The model under review builds one solid part; all positions refer to its coordinate system, in mm. A direction names the side the tool comes from. Round coordinates to 2 decimals unless told otherwise and drop trailing zeros. Order: outer loops, then holes, each group sorted by start corner. A loop starts at its lowest first (then second) coordinate and runs counter-clockwise, first axis right, second up.
Autodesk Inventor part; units mm, degrees
ref_plane "YZ Plane" through (0, 0, 0) normal (1, 0, 0) x (0, 1, 0)
ref_plane "XZ Plane" through (0, 0, 0) normal (0, 1, 0) x (-1, 0, 0)
ref_plane "XY Plane" through (0, 0, 0) normal (0, 0, 1) x (1, 0, 0)
sketch "Sketch1" plane through (0, 0, 0) normal (0, 0, 1) x (1, 0, 0)
  line L0 (-21, 21) -> (21, 21) construction
  line L1 (21, 21) -> (21, -21) construction
  line L2 (21, -21) -> (-21, -21) construction
  line L3 (-21, -21) -> (-21, 21) construction
  line L4 (-21, 16.9706) -> (-21, -16.9706)
  line L5 (-16.9706, -21) -> (16.9706, -21)
  line L6 (21, -16.9706) -> (21, 16.9706)
  line L7 (16.9706, 21) -> (-16.9706, 21)
  arc A0 (-16.9706, 21) -> (-21, 16.9706) centre (0, 0) ccw
  arc A1 (-21, -16.9706) -> (-16.9706, -21) centre (0, 0) ccw
  arc A2 (16.9706, -21) -> (21, -16.9706) centre (0, 0) ccw
  arc A3 (21, 16.9706) -> (16.9706, 21) centre (0, 0) ccw
  dimension "d0" = 42
  dimension "d3" = 27
extrude "Extrusion1" add sketch "Sketch1" along normal blind 11
sketch "Sketch2" plane through (0, 0, 11) normal (0, 0, 1) x (1, 0, 0)
  line L0 (-21, 16.9706) -> (-21, -16.9706)
  arc A0 (-21, -16.9706) -> (-16.9706, -21) centre (0, 0) ccw
  line L1 (-16.9706, -21) -> (16.9706, -21)
  arc A1 (16.9706, -21) -> (21, -16.9706) centre (0, 0) ccw
  line L2 (21, -16.9706) -> (21, 16.9706)
  arc A2 (21, 16.9706) -> (16.9706, 21) centre (0, 0) ccw
  line L3 (16.9706, 21) -> (-16.9706, 21)
  arc A3 (-16.9706, 21) -> (-21, 16.9706) centre (0, 0) ccw
  line L4 (-16.9741, 21.01) -> (16.9741, 21.01)
  arc A4 (21.01, 16.9741) -> (16.9741, 21.01) centre (0, 0) ccw
  line L5 (21.01, 16.9741) -> (21.01, -16.9741)
  arc A5 (16.9741, -21.01) -> (21.01, -16.9741) centre (0, 0) ccw
  line L6 (16.9741, -21.01) -> (-16.9741, -21.01)
  arc A6 (-21.01, -16.9741) -> (-16.9741, -21.01) centre (0, 0) ccw
  line L7 (-21.01, -16.9741) -> (-21.01, 16.9741)
  arc A7 (-16.9741, 21.01) -> (-21.01, 16.9741) centre (0, 0) ccw
  arc A8 (-13.5492, 21.01) -> (-21.01, 13.5492) centre (0, 0) ccw
  arc A9 (-21.01, -13.5492) -> (-13.5492, -21.01) centre (0, 0) ccw
  arc A10 (13.5492, -21.01) -> (21.01, -13.5492) centre (0, 0) ccw
  arc A11 (21.01, 13.5492) -> (13.5492, 21.01) centre (0, 0) ccw
  dimension "d6" = 25
  dimension "d8" = 0.01
extrude "Extrusion2" add sketch "Sketch2" along normal blind 19.116 and the other way blind 2 contours A8 L3 A11 L2 A10 L1 A9 L0 | L0 A9 L7 A8 | A8 L4 A11 L3 | L1 A10 L6 A9 | A11 L5 A10 L2
sketch "Sketch3" plane through (0, 0, 30.116) normal (0, 0, 1) x (1, 0, 0)
  line L0 (-21, 16.9706) -> (-21, -16.9706)
  arc A0 (-16.9706, 21) -> (-21, 16.9706) centre (0, 0) ccw
  line L1 (16.9706, 21) -> (-16.9706, 21)
  arc A1 (21, 16.9706) -> (16.9706, 21) centre (0, 0) ccw
  line L2 (21, -16.9706) -> (21, 16.9706)
  arc A2 (16.9706, -21) -> (21, -16.9706) centre (0, 0) ccw
  line L3 (-16.9706, -21) -> (16.9706, -21)
  arc A3 (-21, -16.9706) -> (-16.9706, -21) centre (0, 0) ccw
extrude "Extrusion3" add sketch "Sketch3" along normal blind 9 and the other way blind 2
sketch "Sketch4" plane through (0, 0, 39.116) normal (0, 0, 1) x (1, 0, 0)
  arc A0 (-16.9706, 21) -> (-21, 16.9706) centre (0, 0) ccw
  circle A1 centre (0, 0) radius 11
  dimension "d17" = 22
extrude "Extrusion4" add sketch "Sketch4" along normal blind 2
sketch "Sketch5" plane through (0, 0, 41.116) normal (0, 0, 1) x (1, 0, 0)
  circle A0 centre (0, 0) radius 11
  circle A1 centre (0, 0) radius 2.5
  dimension "d21" = 5
extrude "Extrusion5" add sketch "Sketch5" along normal blind 22 contours A1
sketch "Sketch6" plane through (0, 0, 63.116) normal (0, 0, 1) x (1, 0, 0)
  circle A0 centre (0, 0) radius 2.5
  line L0 (-1.5, 2) -> (1.5, 2)
  dimension "d25" = 2
extrude "Extrusion6" cut sketch "Sketch6" against normal blind 15 contours L0 A0 picked at (-0.3466, 2.0912)
sketch "Sketch7" plane through (0, 0, 39.116) normal (0, 0, 1) x (1, 0, 0)
  arc A0 (-16.9706, 21) -> (-21, 16.9706) centre (0, 0) ccw
  line L0 (-15.5, 15.5) -> (15.5, 15.5)
  line L1 (15.5, 15.5) -> (15.5, -15.5)
  line L2 (15.5, -15.5) -> (-15.5, -15.5)
  line L3 (-15.5, -15.5) -> (-15.5, 15.5)
  dimension "d28" = 31
hole "Hole1" at (15.5, 15.5, 39.116) at (15.5, -15.5, 39.116) at (-15.5, -15.5, 39.116) at (-15.5, 15.5, 39.116) direction (0, 0, -1) diameter 2.459 depth 10 tip angle 118
properties part number "stepper"
(1) For faces 4 (the flat face through (-18, 18, 28.116)), 5 (the flat face through (-18, -18, 11)), 6 (the cylindrical face through (14.463, 14.839, 34.046)), list the 3-axis set-ups (+Z, -Z, +X, -X, +Y, -Y) from which the entire face can be reached by the end or side of a thin tool; tool diameter is ignored.
Data:
face 4: -X, +Y
face 5: -X, -Y
face 6: +Z
(2) To check wall thickness, follow probe 1 along Y at (x, z) = (-15.5, 36); probe 2 along Y at (x, z) = (15, 33). State the ranges of each line that lie inside material, in increasing order.
Data:
probe 1: y = -21 to -16.73, -14.27 to 14.27, 16.73 to 21
probe 2: y = -21 to -16.62, -14.38 to 14.38, 16.62 to 21
(3) Draft analysis for pull direction X (two halves, no side actions). For faces 1 (the cylindrical face through (-16.537, 14.839, 34.046)), 2 (the flat face through (-21, 0, 35)), 3 (the cylindrical face through (17.625, 17.73, 19.41)), state which applies: pulls with the +X half, pulls with the -X half, needs draft (parallel to the pull), parting line crosses it, or undercut.
Data:
face 1: undercut
face 2: pulls with the -X half
face 3: pulls with the +X half
(4) Consider section A-A (z = 13.5). Write out the cut boundary in (x, y), and give its area (3 significant figures).
Data:
outline: (-21.01, -13.55) arc R25 ccw to (-13.55, -21.01) - (13.55, -21.01) arc R25 ccw to (21.01, -13.55) - (21.01, 13.55) arc R25 ccw to (13.55, 21.01) - (-13.55, 21.01) arc R25 ccw to (-21.01, 13.55) - close
area: 1,670 mm2
(5) Insertion check: pin 1 (3.5 mm diameter, centred on x = 4, z = 6, fed in from +Y); pin 2 (6 mm diameter, centred on x = -18, y = 16.5, fed in from +Z); pin 3 (3 mm diameter, centred on x = -15.5, y = -15.5, fed in from -Z); pin 4 (1.5 mm diameter, centred on x = -4.5, z = 43, fed in from +Y). Each pin has a flat end and moves straight along its axis. Give the tip position at first contact, or say it passes through.
Data:
pin 1: stops at y = 21
pin 2: stops at z = 39.12
pin 3: stops at z = 0
pin 4: passes through
